Check sheet for the drawn part. Datum: minimum x, y, z corner. Units: mm. A direction names the side the tool comes from. Round coordinates to 2 decimals unless told otherwise and drop trailing zeros. Write each loop counter-clockwise with the first axis right and the second up, starting at its lowest first coordinate (ties: lowest second). Pieces come first, ordered by that corner, then holes. Notation, with made-up numbers: M 59.25,6 L 88.25,6 A29 cw 88.25,26 Z; hole C 25.25,34.5 d11. An arc over 180 degrees is marked long. Answer in a Markdown table with one row per item. Add a question column.
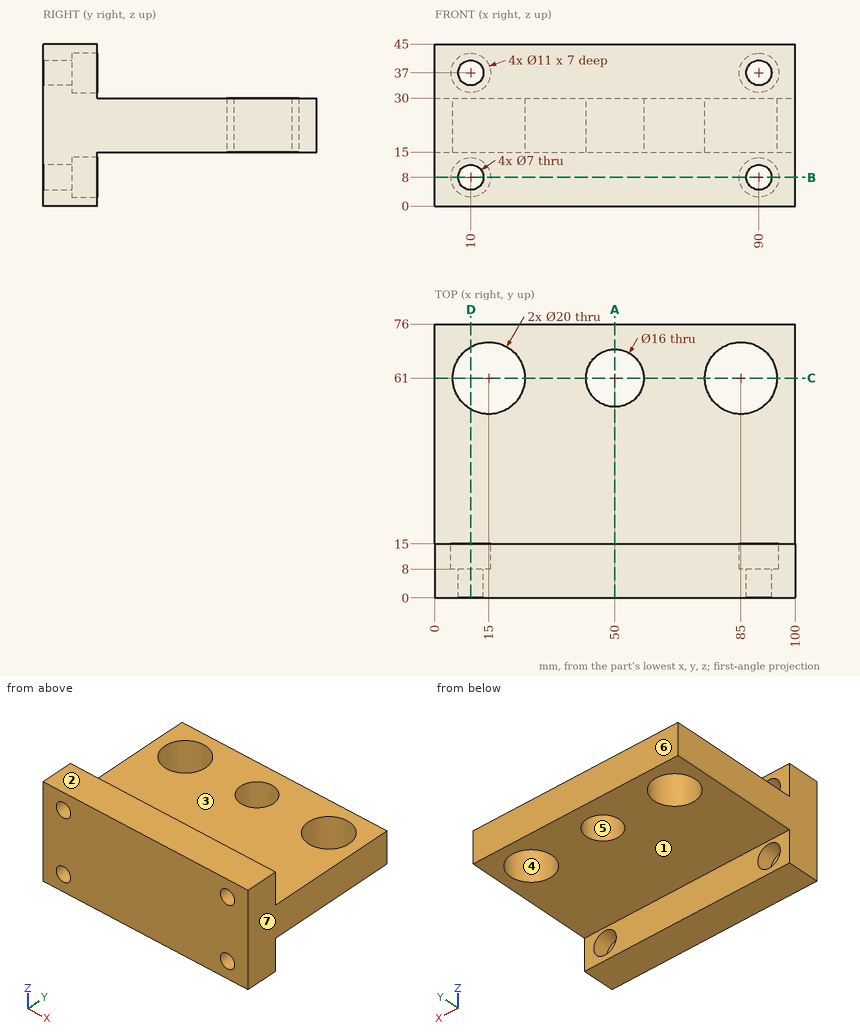
Item 1: Mould release check, pull along Y, two halves, no side actions. Record for the marked faces 4, 5, 6 and 7: +Y half, -Y half, draft (parallel to the pull), parting line (faces both ways), or undercut.
Item 2: Section check A-A, the plane x = 50. Record the boundary of the cut face in (y, z).
Item 3: Section check D-D, the plane x = 10. Record the boundary of the cut face in (y, z).
Item 4: Section check B-B, the plane z = 8. Record the boundary of the cut face in (x, y), and give its area (3 significant figures).
Item 5: Scan lines: probe 1 along X at (y, z) = (11.25, 8); probe 2 along X at (y, z) = (4.75, 37); probe 3 along Y at (x, z) = (85, 24). Record each from-to range of solid material in increasing order. Write a range as from..to.
Item 6: Access from +Z, -Z, +X, -X, +Y, -Y to the whole of each face (thin tool, end or side, straight path). Record for the marked faces 1, 2 and 3.
Item 7: Gauge pin test, flat ends, axial feed: pin 1 Ø1 at (x, y) = (52, 26) entering from +Z; pin 2 Ø5 at (x, y) = (69.5, 56) entering from -Z; pin 3 Ø12 at (x, z) = (90.5, 8) entering from +Y. Record the tip position at first contact, or that the pin passes through.
Item 8: Section check C-C, the plane y = 61. Record the boundary of the cut face in (x, z).
Result sheet:
| question | item | result |
|---|---|---|
| 1 | face 4 | undercut |
| 1 | face 5 | undercut |
| 1 | face 6 | +Y half |
| 1 | face 7 | draft |
| 2 | outline | M 0,0 L 15,0 L 15,15 L 53,15 L 53,30 L 15,30 L 15,45 L 0,45 Z; M 69,15 L 76,15 L 76,30 L 69,30 Z |
| 3 | outline | M 0,0 L 15,0 L 15,2.5 L 8,2.5 L 8,4.5 L 0,4.5 Z; M 0,11.5 L 8,11.5 L 8,13.5 L 15,13.5 L 15,15 L 52.34,15 L 52.34,30 L 15,30 L 15,31.5 L 8,31.5 L 8,33.5 L 0,33.5 Z; M 0,40.5 L 8,40.5 L 8,42.5 L 15,42.5 L 15,45 L 0,45 Z; M 69.66,15 L 76,15 L 76,30 L 69.66,30 Z |
| 4 | outline | M 0,0 L 6.5,0 L 6.5,8 L 4.5,8 L 4.5,15 L 0,15 Z; M 13.5,0 L 86.5,0 L 86.5,8 L 84.5,8 L 84.5,15 L 15.5,15 L 15.5,8 L 13.5,8 Z; M 93.5,0 L 100,0 L 100,15 L 95.5,15 L 95.5,8 L 93.5,8 Z |
| 4 | area | 1,230 mm^2 |
| 5 | probe 1 | x = 0..4.5, 15.5..84.5, 95.5..100 |
| 5 | probe 2 | x = 0..6.5, 13.5..86.5, 93.5..100 |
| 5 | probe 3 | y = 0..51, 71..76 |
| 6 | face 1 | -Z, +X, -X, +Y |
| 6 | face 2 | +Z, +X, -X, +Y, -Y |
| 6 | face 3 | +Z, +X, -X, +Y |
| 7 | pin 1 | stops at z = 30 |
| 7 | pin 2 | stops at z = 15 |
| 7 | pin 3 | stops at y = 15 |
| 8 | outline | M 0,15 L 5,15 L 5,30 L 0,30 Z; M 25,15 L 42,15 L 42,30 L 25,30 Z; M 58,15 L 75,15 L 75,30 L 58,30 Z; M 95,15 L 100,15 L 100,30 L 95,30 Z |
